Input: part model. Units: mm. Frame: model coordinates. A direction names the side the tool comes from. Round coordinates to 2 decimals unless told otherwise and drop trailing zeros. Order: outer loops, then holes, each group sorted by start corner. A loop starts at its lowest first (then second) coordinate and runs counter-clockwise, first axis right, second up. Notation, with made-up numbers: (81, 61) -> (140, 61) arc R18 ccw to (140, 89) -> close; hole circle Ø10 at (53, 24). An arc over 180 degrees is marked (long way). Answer as CSV lines item,"result". Start each with the question number.
1) Section query B-B, the plane y = 0. Output: boundary loops of the cut face in (x, z), and give its area (3 significant figures).
2) First-contact query: P1, Ø3, axis at x = -82.5, y = -11, coming from the -Z side; P2, Ø14, axis at x = -251, y = 15, coming from the -Z side; P3, Ø2.5, axis at x = -254, z = 0, coming from the -Y side. Flat tips, straight axial feed; report the tip coordinate or a pass-through.
3) Section query D-D, the plane y = 44.5. Output: boundary loops of the cut face in (x, z).
4) Line query: L1, parallel to X at y = 20.75, z = 0; L2, parallel to X at y = 11, z = -10.5; L3, parallel to Y at x = -106.5, z = 0. Output: solid intervals per line, ascending.
5) Section query C-C, the plane x = 110.5. Output: boundary loops of the cut face in (y, z), and give its area (3 significant figures).
6) Mould query, pull axis Y, two halves, no side actions, for faces 4 (the face through (-273.14, 45.07, -23.44)), 5 (the face through (-3.91, -6.2, 1.38)), 6 (the face through (266.7, -11, -11)). Classes: +Y half, -Y half, draft (parallel to the pull), parting line (faces both ways), or undercut.
7) Access query for faces 1 (the face through (3.73, -12.4, 2.75)), 2 (the face through (-254, 18, -6.35)), 3 (the face through (-254, 18, 6.35)). Directions: +Z, -Z, +X, -X, +Y, -Y. A direction counts if a zero-diameter tool reaches every point of the face in a straight line with its end or side. Return the directions, or none.
8) Section query A-A, the plane z = -20.5. Output: boundary loops of the cut face in (x, y).
```python
from build123d import *

# Parameters (mm, degrees)
SKETCH1_R                = 12.7
SKETCH1_R_2              = 6.35
BOSS_EXTRUDE1_DEPTH      = 279.4
BOSS_EXTRUDE2_START      = -12.7
SKETCH2_R                = 50.8
SKETCH2_R_2              = 6.35
BOSS_EXTRUDE2_DEPTH      = 12.7
SKETCH3_R                = 50.8
SKETCH3_R_2              = 6.35
BOSS_EXTRUDE3_DEPTH      = 12.7
BOSS_EXTRUDE4_REACH      = 315.889
BOSS_EXTRUDE4_END_RADIUS = 12.7
BOSS_EXTRUDE4_START      = 25.4
SKETCH4_W                = 12.7
SKETCH4_H                = 12.7
SKETCH4_R                = 2.286


with BuildPart() as part:
    # Sketch1 → Boss-Extrude1 (new, symmetric)
    with BuildSketch(Plane(origin=(0, 0, 0), x_dir=(0, 0, -1), z_dir=(1, 0, 0))):
        Circle(SKETCH1_R)
        Circle(SKETCH1_R_2, mode=Mode.SUBTRACT)
    extrude(amount=BOSS_EXTRUDE1_DEPTH, both=True)

    # Sketch2 → Boss-Extrude2 (add)
    with BuildSketch(Plane(origin=(279.4, 0, 0), x_dir=(0, 0, -1), z_dir=(1, 0, 0)).offset(BOSS_EXTRUDE2_START)):
        Circle(SKETCH2_R)
        Circle(SKETCH2_R_2, mode=Mode.SUBTRACT)
    extrude(amount=BOSS_EXTRUDE2_DEPTH)

    # Sketch3 → Boss-Extrude3 (add)
    with BuildSketch(Plane.ZY.offset(279.4)):
        with Locations(Location((0, 0, 0), (0, 0, 180))):
            Circle(SKETCH3_R)
        with Locations(Location((0, 0, 0), (0, 0, 180))):
            Circle(SKETCH3_R_2, mode=Mode.SUBTRACT)
    extrude(amount=-BOSS_EXTRUDE3_DEPTH)

    # Boss-Extrude4: up to this cylinder (the profile starts outside it)
    boss_extrude4_end = Plane(origin=(-254, 0, 0), z_dir=(-1, 0, 0)) * Cylinder(BOSS_EXTRUDE4_END_RADIUS, 658.178, mode=Mode.PRIVATE)
    # Sketch4 → Boss-Extrude4 (add, up to the surface)
    with BuildSketch(Plane(origin=(0, 0, 0), x_dir=(1, 0, 0), z_dir=(0, 1, 0)).offset(BOSS_EXTRUDE4_START), mode=Mode.PRIVATE) as boss_extrude4_sk1:
        with Locations((-254, 0)):
            Rectangle(SKETCH4_W, SKETCH4_H)
        with Locations(Location((-254, 0, 0), (0, 0, 270))):
            Circle(SKETCH4_R, mode=Mode.SUBTRACT)
    boss_extrude4_tool1 = extrude(boss_extrude4_sk1.sketch, amount=-BOSS_EXTRUDE4_REACH, mode=Mode.PRIVATE) - boss_extrude4_end
    add(boss_extrude4_tool1.solids().sort_by_distance((-254, 25.4, 6.170395))[0])


solid = part.part
```
Findings:
1,outline,"(-279.4, -50.8) -> (-266.7, -50.8) -> (-266.7, -12.7) -> (266.7, -12.7) -> (266.7, -50.8) -> (279.4, -50.8) -> (279.4, -6.35) -> (-279.4, -6.35) -> close; (-279.4, 6.35) -> (279.4, 6.35) -> (279.4, 50.8) -> (266.7, 50.8) -> (266.7, 12.7) -> (-266.7, 12.7) -> (-266.7, 50.8) -> (-279.4, 50.8) -> close"
1,area,"9,030 mm^2"
2,P1,"stops at z = -8.43"
2,P2,"stops at z = -9.86"
2,P3,"stops at y = -12.7"
3,outline,"(-279.4, -24.5) -> (-266.7, -24.5) -> (-266.7, 24.5) -> (-279.4, 24.5) -> close; (266.7, -24.5) -> (279.4, -24.5) -> (279.4, 24.5) -> (266.7, 24.5) -> close"
4,L1,"x = -279.4 to -266.7, -260.35 to -256.29, -251.71 to -247.65, 266.7 to 279.4"
4,L2,"x = -279.4 to -266.7, 266.7 to 279.4"
4,L3,"y = -12.7 to -6.35, 6.35 to 12.7"
5,outline,"circle Ø25.4 at (0, 0); hole circle Ø12.7 at (0, 0)"
5,area,"380 mm^2"
6,face 4,"parting line"
6,face 5,"undercut"
6,face 6,"draft"
7,face 1,"none"
7,face 2,"-Z, +Y"
7,face 3,"+Z, +Y"
8,outline,"(-279.4, -46.48) -> (-266.7, -46.48) -> (-266.7, 46.48) -> (-279.4, 46.48) -> close; (266.7, -46.48) -> (279.4, -46.48) -> (279.4, 46.48) -> (266.7, 46.48) -> close"
